The model under review builds one solid part; all positions refer to its coordinate system, in mm. A direction names the side the tool comes from. Give positions to 0.01 mm unless a question says otherwise; leave off trailing zeros. Loops run counter-clockwise (first coordinate to the right, second up) from the corner with the lowest first, then second, coordinate; pieces in that order, holes last. Notation, with made-up numbers: (16.5, 53) -> (39.5, 53) arc R22 cw to (39.5, 77) -> close; hole circle Ø8 at (78, 75.25). An arc over 180 degrees is marked (long way). Write each question's results on one line, items separated by ' | '. Start each with the question number.
Q1. We need section D-D (z = 1). Write out the cut boundary in (x, y) (3 decimals).
Q2. We need section A-A (x = 23.5). Write out the cut boundary in (y, z).
Q3. Machinability: for faces 1 (the face through (21, -33.91, 1)), 2 (the face through (4, -13.26, 2)), 3 (the face through (-3.924, -22, 2)), 4 (the face through (-14.224, -38, 1)), 5 (the face through (4, -30.26, 2)), which of the approach directions +Z, -Z, +X, -X, +Y, -Y give a long, thin tool a straight path to every point of the face, cutting with its end or side? Answer none if there is none.
Q4. Mouldability with a two-part tool opening along Y and no side actions: class faces 6 (the face through (0, -15, 0)), 7 (the face through (11.23, -35.8, 0.79)), 8 (the face through (-21, -33.91, 1)), 9 (the face through (-24.96, -26.71, 0.79)) as released by +Y, released by -Y, zero draft, split by the parting line, or undercut.
Q5. We need section C-C (y = -22). Write out the cut boundary in (x, z).
Q6. Wall thickness on L1, parallel to Y at x = -21.5, z = 1.4; L2, parallel to Y at x = -2, z = 1.75; L3, parallel to X at y = 8.5, z = 1.4: over which ranges is each line inside the solid? List them lowest first. Write a range as [from, to].
Q7. Insertion check: pin 1 Ø0.5 at (y, z) = (-36.5, 1) entering from +X; pin 2 Ø1.8 at (x, z) = (-20.5, 0.5) entering from -Y; pin 3 Ø3.5 at (x, y) = (-10.414, -37.085) entering from +Z. Each pin has a flat end and moves straight along its axis. Give the tip position at first contact, or say it passes through.
Q8. We need section B-B (x = -23). Write out the cut boundary in (y, z).
from build123d import *

# Parameters (mm, degrees)
EXTRUDE1_DEPTH = 1.6
SKETCH2_R      = 1.524
EXTRUDE2_DEPTH = 2.6
SKETCH4_W      = 17
SKETCH4_H      = 17
EXTRUDE3_DEPTH = 1.6


with BuildPart() as part:
    # Sketch1 → Extrude1 (new body)
    with BuildSketch(Plane.XY):
        Polygon((15.724, -33.91), (26.924, -33.91), (26.924, 10.54), (-26.924, 10.54), (-26.924, -33.91), (-15.724, -33.91), (-14.224, -35.41), (-14.224, -40.26), (14.224, -40.26), (14.224, -35.41), align=None)
    extrude(amount=EXTRUDE1_DEPTH)

    # Sketch2 → Extrude2 (cut, through all)
    with BuildSketch(Plane.XY):
        with Locations((23.749, 7.365)):
            Circle(SKETCH2_R)
        with Locations((10.414, -37.085)):
            Circle(SKETCH2_R)
        with Locations((-10.414, -37.085)):
            Circle(SKETCH2_R)
        with Locations((-23.749, -25.782)):
            Circle(SKETCH2_R)
        with Locations((-23.749, 7.365)):
            Circle(SKETCH2_R)
    extrude(amount=EXTRUDE2_DEPTH, mode=Mode.SUBTRACT)

    # Sketch4 → Extrude3 (add)
    with BuildSketch(Plane.XY.offset(1.6)):
        with Locations((4.576, -21.76)):
            Rectangle(SKETCH4_W, SKETCH4_H)
    extrude(amount=EXTRUDE3_DEPTH)


solid = part.part
Output:
1) outline: (-26.924, -33.91) -> (-15.724, -33.91) -> (-14.224, -35.41) -> (-14.224, -40.26) -> (14.224, -40.26) -> (14.224, -35.41) -> (15.724, -33.91) -> (26.924, -33.91) -> (26.924, 10.54) -> (-26.924, 10.54) -> close; hole circle Ø3.048 at (-23.749, -25.782); hole circle Ø3.048 at (-23.749, 7.365); hole circle Ø3.048 at (-10.414, -37.085); hole circle Ø3.048 at (10.414, -37.085); hole circle Ø3.048 at (23.749, 7.365)
2) outline: (-33.91, 0) -> (5.86, 0) -> (5.86, 1.6) -> (-33.91, 1.6) -> close; (8.87, 0) -> (10.54, 0) -> (10.54, 1.6) -> (8.87, 1.6) -> close
3) face 1: +Z, -Z, +X, -Y | face 2: +Z, +X, -X, +Y | face 3: +Z, -X, +Y, -Y | face 4: +Z, -Z, -X, -Y | face 5: +Z, +X, -X, -Y
4) face 6: zero draft | face 7: undercut | face 8: released by -Y | face 9: undercut
5) outline: (-26.92, 0) -> (26.92, 0) -> (26.92, 1.6) -> (13.08, 1.6) -> (13.08, 3.2) -> (-3.92, 3.2) -> (-3.92, 1.6) -> (-26.92, 1.6) -> close
6) L1: [-33.91, 10.54] | L2: [-30.26, -13.26] | L3: [-26.92, -24.77], [-22.73, 22.73], [24.77, 26.92]
7) pin 1: x = 14.22 | pin 2: y = -33.91 | pin 3: z = 1.6
8) outline: (-33.91, 0) -> (-27.11, 0) -> (-27.11, 1.6) -> (-33.91, 1.6) -> close; (-24.45, 0) -> (6.04, 0) -> (6.04, 1.6) -> (-24.45, 1.6) -> close; (8.69, 0) -> (10.54, 0) -> (10.54, 1.6) -> (8.69, 1.6) -> close
